Verification items for the finished model (mm, model axes). Round coordinates to 2 decimals unless told otherwise and drop trailing zeros. Order: outer loops, then holes, each group sorted by start corner. A loop starts at its lowest first (then second) coordinate and runs counter-clockwise, first axis right, second up. Notation, with made-up numbers: M -14,-4.5 L 9,-4.5 A6 cw 9,6.5 Z; hole C -19.75,73 d2. An arc over 180 degrees is marked long. Use CSV: the item, a comma, the result in double quotes. Start each with the question number.
Q1. Sectioned sample at C-C (y = -7.5). Enter the section's corners in (x, z), and give its area (3 significant figures).
Q2. Scan lines: line 1 (X direction, y = 35, z = 0.2); line 2 (Y direction, x = 250.5, z = 0.5); line 3 (Y direction, x = 269, z = 0.8). Record each from-to range of solid material in increasing order.
Q3. Sectioned sample at B-B (z = 0.45). State how many separate pieces and enclosed holes the cut face has, and give its area (3 significant figures).
Q4. Gauge pin test, flat ends, axial feed: pin 1 Ø0.5 at (x, z) = (313.5, 1) entering from +Y; pin 2 Ø0.8 at (y, z) = (61, 1) entering from -X. Record the tip position at first contact, or that the pin passes through.
Q5. Sectioned sample at A-A (x = 264.5). Enter the section's corners in (y, z), and give its area (3 significant figures).
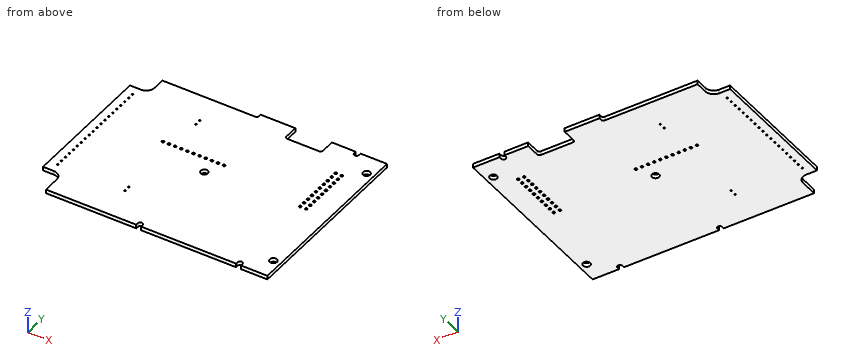
```python
from build123d import *

# Parameters (mm, degrees)
BOSS_EXTRUDE1_DEPTH = 1.6
SKETCH3_R           = 1.5
CUT_EXTRUDE1_DEPTH  = 2.6
SKETCH4_W           = 50
SKETCH4_H           = 85
CUT_EXTRUDE2_DEPTH  = 2.6
SKETCH5_R           = 0.3
CUT_EXTRUDE3_DEPTH  = 2.6
SKETCH6_R           = 0.499999
CUT_EXTRUDE4_DEPTH  = 2.6
SKETCH7_R           = 0.499999
CUT_EXTRUDE5_DEPTH  = 2.6


with BuildPart() as part:
    # Board Outline → Boss-Extrude1 (new body)
    with BuildSketch(Plane.XY):
        with BuildLine():
            Line((394.450402667, 53.680474091), (394.450402667, -2.319525909))
            Line((394.450402667, -2.319525909), (375.450402667, -2.319525909))
            ThreePointArc((375.450402667, -2.319525909), (372.975528933, -3.344652175), (371.950402667, -5.819525909))
            Line((371.950402667, -5.819525909), (371.950402667, -12.819525909))
            Line((371.950402667, -12.819525909), (334.950402667, -12.819525909))
            Line((334.950402667, -12.819525909), (334.950402667, -11.819525909))
            ThreePointArc((334.950402667, -11.819525909), (333.950402667, -10.819525909), (332.950402667, -11.819525909))
            Line((332.950402667, -11.819525909), (332.950402667, -12.819525909))
            Line((332.950402667, -12.819525909), (293.450402667, -12.819525909))
            Line((293.450402667, -12.819525909), (293.450402667, -11.819525909))
            ThreePointArc((293.450402667, -11.819525909), (292.450402667, -10.819525909), (291.450402667, -11.819525909))
            Line((291.450402667, -11.819525909), (291.450402667, -12.819525909))
            Line((291.450402667, -12.819525909), (253.950402667, -12.819525909))
            Line((253.950402667, -12.819525909), (253.950402667, -5.819525909))
            ThreePointArc((253.950402667, -5.819525909), (252.925276401, -3.344652175), (250.450402667, -2.319525909))
            Line((250.450402667, -2.319525909), (245.950402667, -2.319525909))
            Line((245.950402667, -2.319525909), (245.950402667, 53.680474091))
            Line((245.950402667, 53.680474091), (250.450402667, 53.680474091))
            ThreePointArc((250.450402667, 53.680474091), (252.925276401, 54.705600357), (253.950402667, 57.180474091))
            Line((253.950402667, 57.180474091), (253.950402667, 62.180474091))
            Line((253.950402667, 62.180474091), (292.450402667, 62.180474091))
            ThreePointArc((292.450402667, 62.180474091), (293.157509449, 62.47336731), (293.450402667, 63.180474091))
            Line((293.450402667, 63.180474091), (293.450402667, 64.180474091))
            Line((293.450402667, 64.180474091), (307.850402667, 64.180474091))
            Line((307.850402667, 64.180474091), (307.850402667, 58.480474091))
            ThreePointArc((307.850402667, 58.480474091), (308.143295886, 57.77336731), (308.850402667, 57.480474091))
            Line((308.850402667, 57.480474091), (322.050402667, 57.480474091))
            ThreePointArc((322.050402667, 57.480474091), (322.757509449, 57.77336731), (323.050402667, 58.480474091))
            Line((323.050402667, 58.480474091), (323.050402667, 64.180474091))
            Line((323.050402667, 64.180474091), (332.950402667, 64.180474091))
            Line((332.950402667, 64.180474091), (332.950402667, 63.180474091))
            ThreePointArc((332.950402667, 63.180474091), (333.950402667, 62.180474091), (334.950402667, 63.180474091))
            Line((334.950402667, 63.180474091), (334.950402667, 64.180474091))
            Line((334.950402667, 64.180474091), (371.950402667, 64.180474091))
            Line((371.950402667, 64.180474091), (371.950402667, 57.180474091))
            ThreePointArc((371.950402667, 57.180474091), (372.975528933, 54.705600357), (375.450402667, 53.680474091))
            Line((375.450402667, 53.680474091), (394.450402667, 53.680474091))
        make_face()
    extrude(amount=BOSS_EXTRUDE1_DEPTH)

    # Sketch3 → Cut-Extrude1 (cut, through all)
    with BuildSketch(Plane.XY.offset(1.6)):
        with Locations((294.950402667, 25.680474091)):
            Circle(SKETCH3_R)
        with Locations((342.950402667, -4.319525909)):
            Circle(SKETCH3_R)
        with Locations((342.950402667, 55.680474091)):
            Circle(SKETCH3_R)
    extrude(amount=-CUT_EXTRUDE1_DEPTH, mode=Mode.SUBTRACT)

    # Sketch4 → Cut-Extrude2 (cut, through all)
    with BuildSketch(Plane.XY.offset(1.6)):
        with Locations((370.950402667, 25.680474091)):
            Rectangle(SKETCH4_W, SKETCH4_H)
    extrude(amount=-CUT_EXTRUDE2_DEPTH, mode=Mode.SUBTRACT)

    # Sketch5 → Cut-Extrude3 (cut, through all)
    with BuildSketch(Plane.XY.offset(1.6)):
        with Locations((249.525402667, 49.810474091)):
            Circle(SKETCH5_R)
        with Locations((277.475402667, 49.810474091)):
            Circle(SKETCH5_R)
        with Locations((277.475402667, 47.270474091)):
            Circle(SKETCH5_R)
        with Locations((277.475402667, 4.090474091)):
            Circle(SKETCH5_R)
        with Locations((249.525402667, 47.270474091)):
            Circle(SKETCH5_R)
        with Locations((249.525402667, 44.730474091)):
            Circle(SKETCH5_R)
        with Locations((249.525402667, 42.190474091)):
            Circle(SKETCH5_R)
        with Locations((249.525402667, 39.650474091)):
            Circle(SKETCH5_R)
        with Locations((249.525402667, 37.110474091)):
            Circle(SKETCH5_R)
        with Locations((249.525402667, 34.570474091)):
            Circle(SKETCH5_R)
        with Locations((249.525402667, 32.030474091)):
            Circle(SKETCH5_R)
        with Locations((249.525402667, 29.490474091)):
            Circle(SKETCH5_R)
        with Locations((249.525402667, 26.950474091)):
            Circle(SKETCH5_R)
        with Locations((249.525402667, 24.410474091)):
            Circle(SKETCH5_R)
        with Locations((249.525402667, 21.870474091)):
            Circle(SKETCH5_R)
        with Locations((249.525402667, 19.330474091)):
            Circle(SKETCH5_R)
        with Locations((249.525402667, 16.790474091)):
            Circle(SKETCH5_R)
        with Locations((249.525402667, 14.250474091)):
            Circle(SKETCH5_R)
        with Locations((249.525402667, 11.710474091)):
            Circle(SKETCH5_R)
        with Locations((249.525402667, 9.170474091)):
            Circle(SKETCH5_R)
        with Locations((249.525402667, 6.630474091)):
            Circle(SKETCH5_R)
        with Locations((249.525402667, 4.090474091)):
            Circle(SKETCH5_R)
        with Locations((249.525402667, 1.550474091)):
            Circle(SKETCH5_R)
        with Locations((277.475402667, 1.550474091)):
            Circle(SKETCH5_R)
    extrude(amount=-CUT_EXTRUDE3_DEPTH, mode=Mode.SUBTRACT)

    # Sketch6 → Cut-Extrude4 (cut, through all)
    with BuildSketch(Plane(origin=(0, 0, 0), x_dir=(-1, 0, 0), z_dir=(0, 0, -1))):
        with Locations((-333.834418667, 49.903457691)):
            Circle(SKETCH6_R)
        with Locations((-333.834418667, 47.363457691)):
            Circle(SKETCH6_R)
        with Locations((-336.374418667, 47.363457691)):
            Circle(SKETCH6_R)
        with Locations((-336.374418667, 44.823457691)):
            Circle(SKETCH6_R)
        with Locations((-333.834418667, 44.823457691)):
            Circle(SKETCH6_R)
        with Locations((-333.834418667, 34.663457691)):
            Circle(SKETCH6_R)
        with Locations((-333.834418667, 37.203457691)):
            Circle(SKETCH6_R)
        with Locations((-333.834418667, 39.743457691)):
            Circle(SKETCH6_R)
        with Locations((-333.834418667, 42.283457691)):
            Circle(SKETCH6_R)
        with Locations((-336.374418667, 42.283457691)):
            Circle(SKETCH6_R)
        with Locations((-336.374418667, 39.743457691)):
            Circle(SKETCH6_R)
        with Locations((-336.374418667, 37.203457691)):
            Circle(SKETCH6_R)
        with Locations((-333.834418667, 32.123457691)):
            Circle(SKETCH6_R)
        with Locations((-336.374418667, 34.663457691)):
            Circle(SKETCH6_R)
        with Locations((-336.374418667, 32.123457691)):
            Circle(SKETCH6_R)
        with Locations((-333.834418667, 29.583457691)):
            Circle(SKETCH6_R)
        with Locations((-336.374418667, 27.043457691)):
            Circle(SKETCH6_R)
        with Locations((-333.834418667, 27.043457691)):
            Circle(SKETCH6_R)
        with Locations((-336.374418667, 29.583457691)):
            Circle(SKETCH6_R)
        with Locations((-336.374418667, 49.903457691)):
            Circle(SKETCH6_R)
    extrude(amount=-CUT_EXTRUDE4_DEPTH, mode=Mode.SUBTRACT)

    # Sketch7 → Cut-Extrude5 (cut, through all)
    with BuildSketch(Plane.XY.offset(1.6)):
        with Locations((298.650402667, 32.616474091)):
            Circle(SKETCH7_R)
        with Locations((296.110402667, 32.616474091)):
            Circle(SKETCH7_R)
        with Locations((293.570402667, 32.616474091)):
            Circle(SKETCH7_R)
        with Locations((291.030402667, 32.616474091)):
            Circle(SKETCH7_R)
        with Locations((288.490402667, 32.616474091)):
            Circle(SKETCH7_R)
        with Locations((285.950402667, 32.616474091)):
            Circle(SKETCH7_R)
        with Locations((283.410402667, 32.616474091)):
            Circle(SKETCH7_R)
        with Locations((280.870402667, 32.616474091)):
            Circle(SKETCH7_R)
        with Locations((278.330402667, 32.616474091)):
            Circle(SKETCH7_R)
        with Locations((275.790402667, 32.616474091)):
            Circle(SKETCH7_R)
        with Locations((273.250402667, 32.616474091)):
            Circle(SKETCH7_R)
    extrude(amount=-CUT_EXTRUDE5_DEPTH, mode=Mode.SUBTRACT)


solid = part.part
```
Verdict:
1,outline,"M 253.95,0 L 345.95,0 L 345.95,1.6 L 253.95,1.6 Z"
1,area,"147 mm²"
2,line 1,"x = 245.95 to 333.46, 334.2 to 336, 336.74 to 345.95"
2,line 2,"y = -2.32 to 53.68"
2,line 3,"y = -12.82 to 62.18"
3,separate pieces,"1"
3,enclosed holes,"58"
3,area,"7,290 mm²"
4,pin 1,"stops at y = 57.48"
4,pin 2,"stops at x = 253.95"
5,outline,"M -12.82,0 L 62.18,0 L 62.18,1.6 L -12.82,1.6 Z"
5,area,"120 mm²"
